Read the model definition and answer for the solid it produces. Units are mm, in the model's axes. A direction names the side the tool comes from. Give positions to 0.01 mm unless a question says otherwise; leave off trailing zeros. Loops run counter-clockwise (first coordinate to the right, second up) from the corner with the lowest first, then second, coordinate; pieces in that order, holes last. Notation, with made-up numbers: (78, 87) - (103, 87) arc R35 ccw to (103, 122) - close; hole circle Ø3 at (21, 49.5). An arc over 180 degrees is marked (long way). Write item = value, one per line.
```python
from build123d import *

# Parameters (mm, degrees)
SKETCH1_R           = 15
BOSS_EXTRUDE1_DEPTH = 23
SKETCH1_3_R         = 15
SKETCH1_3_R_2       = 6
BOSS_EXTRUDE2_DEPTH = 3
CUT_EXTRUDE1_REACH  = 181.569
SKETCH2_W           = 16
SKETCH2_H           = 12
CUT_EXTRUDE2_REACH  = 181.569
SKETCH3_R           = 3


with BuildPart() as part:
    # Sketch1 → Boss-Extrude1 (new body)
    with BuildSketch(Plane.XY):
        Polygon((0, 150), (0, 98), (68, 98), (68, 0), (96, 0), (96, 150), align=None)
        with Locations((23, 124)):
            Circle(SKETCH1_R, mode=Mode.SUBTRACT)
    extrude(amount=BOSS_EXTRUDE1_DEPTH)

    # Sketch1_3 → Boss-Extrude2 (add)
    with BuildSketch(Plane.XY):
        with Locations((23, 124)):
            Circle(SKETCH1_3_R)
        with Locations((23, 124)):
            Circle(SKETCH1_3_R_2, mode=Mode.SUBTRACT)
    extrude(amount=BOSS_EXTRUDE2_DEPTH)

    # Sketch2 → Cut-Extrude1 (cut, up to next)
    with BuildSketch(Plane(origin=(0, 150, 0), x_dir=(1, 0, 0), z_dir=(0, 1, 0)), mode=Mode.PRIVATE) as cut_extrude1_sk1:
        with Locations((8, -11.5)):
            Rectangle(SKETCH2_W, SKETCH2_H)
    cut_extrude1_tool1 = extrude(cut_extrude1_sk1.sketch, amount=-CUT_EXTRUDE1_REACH, mode=Mode.PRIVATE) & part.part
    add(cut_extrude1_tool1.solids().sort_by_distance((8, 150, 11.5))[0], mode=Mode.SUBTRACT)

    # Sketch3 → Cut-Extrude2 (cut, up to next)
    with BuildSketch(Plane(origin=(96, 0, 0), x_dir=(0, 0, -1), z_dir=(1, 0, 0)), mode=Mode.PRIVATE) as cut_extrude2_sk1:
        with Locations((-11.5, 12)):
            Circle(SKETCH3_R)
    cut_extrude2_tool1 = extrude(cut_extrude2_sk1.sketch, amount=-CUT_EXTRUDE2_REACH, mode=Mode.PRIVATE) & part.part
    add(cut_extrude2_tool1.solids().sort_by_distance((96, 12, 11.5))[0], mode=Mode.SUBTRACT)


solid = part.part
```
1) A cutting plane is placed at A-A on x = 23. Determine the outline of the cut face in (y, z).
Output:
outline = (98, 0) - (118, 0) - (118, 3) - (109, 3) - (109, 23) - (98, 23) - close; (130, 0) - (150, 0) - (150, 23) - (139, 23) - (139, 3) - (130, 3) - close
2) Find the intervals of material crossed by probe 1 along X at (y, z) = (124, 19); probe 2 along Y at (x, z) = (23, 1.75); probe 3 along Y at (x, z) = (86.5, 11.5), in increasing order.
Output:
probe_1 = 0 to 8, 38 to 96
probe_2 = 98 to 118, 130 to 150
probe_3 = 0 to 9, 15 to 150
3) Each of these flat-tipped pins is pushed along its axis until it touches: P1, Ø18, axis at x = 23, y = 124, coming from the +Z side; P2, Ø5, axis at x = 56, z = 15, coming from the -Y side; P3, Ø7, axis at y = 12, z = 11.5, coming from the -X side. Where does it stop, or does it pass through?
Output:
P1 = 3
P2 = 98
P3 = 68
4) The mould has two halves that part along Y. Classify faces 1 (the face through (49, 150, 11)), 2 (the face through (18.58, 128.06, 1.48)), 3 (the face through (69, 93, 23)): pulls with the +Y half, pulls with the -Y half, needs draft (parallel to the pull), parting line crosses it, or undercut.
Output:
face_1 = pulls with the +Y half
face_2 = undercut
face_3 = needs draft
5) A cutting plane is placed at D-D on z = 19.25. Determine the outline of the cut face in (x, y).
Output:
outline = (0, 98) - (68, 98) - (68, 0) - (96, 0) - (96, 150) - (0, 150) - close; hole circle Ø30 at (23, 124)
6) A cutting plane is placed at B-B on z = 11.5. Determine the outline of the cut face in (x, y), then the cut area to 3 significant figures.
Output:
outline = (16, 98) - (68, 98) - (68, 15) - (96, 15) - (96, 150) - (16, 150) - (16, 137.27) arc R15 cw (long way) to (16, 110.73) - close; (68, 0) - (96, 0) - (96, 9) - (68, 9) - close
area = 6,180 mm²
7) A cutting plane is placed at C-C on y = 12. Determine the outline of the cut face in (x, z), then the cut area to 3 significant figures.
Output:
outline = (68, 0) - (96, 0) - (96, 8.5) - (68, 8.5) - close; (68, 14.5) - (96, 14.5) - (96, 23) - (68, 23) - close
area = 476 mm²
8) A tool of negligible diameter and unlimited length cuts with its end or side. For faces 4 (the face through (29.5, 124.2, 3)), 5 (the face through (68, 50, 11)), 6 (the face through (82.2, 10.2, 13.9)), 7 (the face through (82, 0, 11)), 8 (the face through (16, 104, 12)), from which of +Z, -Z, +X, -X, +Y, -Y can it reach the whole face along a straight path? Write none if from no direction.
Output:
face_4 = +Z
face_5 = +Z, -Z, -X, -Y
face_6 = +X, -X
face_7 = +Z, -Z, +X, -X, -Y
face_8 = -X, +Y, -Y
